Autodesk Inventor part; units mm, degrees
ref_plane "YZ Plane" through (0, 0, 0) normal (1, 0, 0) x (0, 1, 0)
ref_plane "XZ Plane" through (0, 0, 0) normal (0, 1, 0) x (-1, 0, 0)
ref_plane "XY Plane" through (0, 0, 0) normal (0, 0, 1) x (1, 0, 0)
sketch "Sketch1" plane through (0, 0, 0) normal (0, 1, 0) x (-1, 0, 0)
  line L0 (32.6378, 42.945) -> (-32.3622, 42.945)
  line L1 (32.6378, 42.945) -> (32.6378, -42.055)
  line L2 (32.6378, -42.055) -> (-32.3622, -42.055)
  line L3 (-32.3622, -42.055) -> (-32.3622, 42.945)
  line L4 (-34.8622, 45.445) -> (35.1378, 45.445)
  line L5 (35.1378, -44.555) -> (-34.8622, -44.555)
  line L6 (35.1378, -44.555) -> (35.1378, 45.445)
  line L7 (-34.8622, -44.555) -> (-34.8622, 45.445)
  point P0 (0, 0)
  dimension "d0" = 65
  dimension "d1" = 85
  dimension "d6" = 70
  dimension "d7" = 90
extrude "Extrusion1" add sketch "Sketch1" along normal blind 2 contours L1 L2 L3 L0
extrude "Extrusion2" add sketch "Sketch1" along normal blind 5.5
sketch "Sketch2" plane through (0, 2, 0) normal (0, 1, 0) x (1, 0, 0)
  line L0 (32.3622, 42.055) -> (-32.6378, 42.055)
  line L1 (13.6122, 31.055) -> (13.6122, 11.855)
  line L2 (13.6122, 11.855) -> (-13.8878, 11.855)
  line L3 (-13.8878, 11.855) -> (-13.8878, 31.055)
  line L4 (-13.8878, 31.055) -> (13.6122, 31.055)
  point P0 (0, 0)
  dimension "d15" = 19.2
  dimension "d16" = 27.5
extrude "Extrusion3" cut sketch "Sketch2" against normal blind 5
properties part number "Tampa"
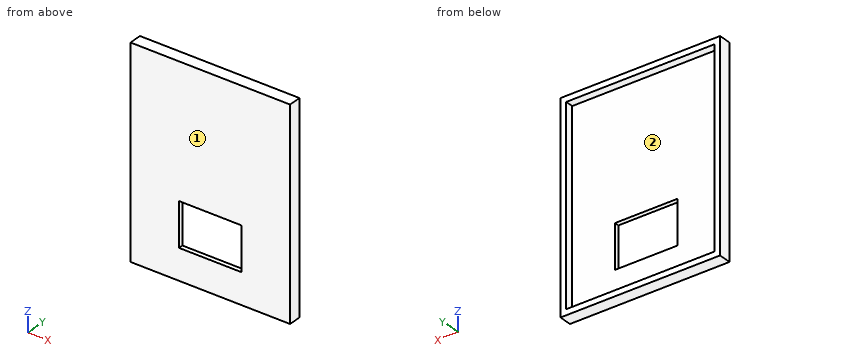
For this review, take the finished solid that the model builds, in its own axes (mm). Face numbers are marked on the shaded views. Give positions to 0.01 mm unless a question says otherwise; leave off trailing zeros. Order: outer loops, then holes, each group sorted by start corner. A loop starts at its lowest first (then second) coordinate and runs counter-clockwise, first axis right, second up. Notation, with made-up numbers: M 74,45.5 L 108,45.5 A12 cw 108,50.5 Z; hole C 33.25,-33.5 d4. An arc over 180 degrees is marked long. Answer in a Markdown table with one row per item. Add a question column.
(1) Consider section D-D on x = -19.5. State the section outline as (y, z) points (3 decimals), and give its area (4 significant figures).
(2) Wall thickness on probe 1 along X at (y, z) = (4.95, -12.5); probe 2 along X at (y, z) = (0.5, -16); probe 3 along Z at (x, y) = (18, 3.5) (3 decimals): over which ranges is each line inside the solid? List them lowest first. Write a range as [from, to].
(3) For pin 1 (10 mm diameter, centred on x = 23.5, z = 10, fed in from +Y), flat-tipped, find the tip position at first contact; note if it passes through.
(4) Consider section C-C on z = 8.5. State the section outline as (x, y) points.
(5) Mouldability with a two-part tool opening along Z and no side actions: class the marked faces 1 and 2 as +Z half, -Z half, draft (parallel to the pull), parting line (faces both ways), or undercut.
(6) Consider section B-B on y = 1. State the section outline as (x, z) points (3 decimals).
(7) Consider section A-A on x = 6.5. State the section outline as (y, z) points (3 decimals).
Evaluation:
| question | item | result |
|---|---|---|
| 1 | outline | M 0,-44.555 L 5.5,-44.555 L 5.5,-42.055 L 2,-42.055 L 2,42.945 L 5.5,42.945 L 5.5,45.445 L 0,45.445 Z |
| 1 | area | 197.5 mm^2 |
| 2 | probe 1 | x = [-35.14, -32.64], [32.36, 34.86] |
| 2 | probe 2 | x = [-35.14, -13.89], [13.61, 34.86] |
| 2 | probe 3 | z = [-44.555, -42.055], [42.945, 45.445] |
| 3 | pin 1 | stops at y = 2 |
| 4 | outline | M -35.14,0 L 34.86,0 L 34.86,5.5 L 32.36,5.5 L 32.36,2 L -32.64,2 L -32.64,5.5 L -35.14,5.5 Z |
| 5 | face 1 | draft |
| 5 | face 2 | undercut |
| 6 | outline | M -35.138,-44.555 L 34.862,-44.555 L 34.862,45.445 L -35.138,45.445 Z; hole M -13.888,-31.055 L 13.612,-31.055 L 13.612,-11.855 L -13.888,-11.855 Z |
| 7 | outline | M 0,-44.555 L 5.5,-44.555 L 5.5,-42.055 L 2,-42.055 L 2,-31.055 L 0,-31.055 Z; M 0,-11.855 L 2,-11.855 L 2,42.945 L 5.5,42.945 L 5.5,45.445 L 0,45.445 Z |
